```python
from build123d import *

# Parameters (mm, degrees)
ESQUISSE1_W        = 16
ESQUISSE1_H        = 28
BOSS_EXTRU_1_DEPTH = 6
BOSS_EXTRU_2_DEPTH = 0.5
CONG_1_R           = 0.5
ESQUISSE3_W        = 1
ESQUISSE3_H        = 4.650680728
BOSS_EXTRU_3_DEPTH = 0.5
ESQUISSE4_W        = 1
ESQUISSE4_H        = 3.990373045
BOSS_EXTRU_4_DEPTH = 0.5


with BuildPart() as part:
    # Esquisse1 → Boss.-Extru.1 (new body)
    with BuildSketch(Plane.XY):
        with Locations((2.66318356, 3.111111111)):
            Rectangle(ESQUISSE1_W, ESQUISSE1_H)
    extrude(amount=BOSS_EXTRU_1_DEPTH)

    # Esquisse2 → Boss.-Extru.2 (add)
    with BuildSketch(Plane.XY.offset(6)):
        with BuildLine():
            Line((-2.33681644, -0.888888889), (7.66318356, -0.888888889))
            ThreePointArc((7.66318356, -0.888888889), (8.370290341, -1.181782108), (8.66318356, -1.888888889))
            Line((8.66318356, -1.888888889), (8.66318356, -5.388888889))
            ThreePointArc((8.66318356, -5.388888889), (8.370290341, -6.09599567), (7.66318356, -6.388888889))
            Line((7.66318356, -6.388888889), (-2.33681644, -6.388888889))
            ThreePointArc((-2.33681644, -6.388888889), (-3.043923221, -6.09599567), (-3.33681644, -5.388888889))
            Line((-3.33681644, -5.388888889), (-3.33681644, -1.888888889))
            ThreePointArc((-3.33681644, -1.888888889), (-3.043923221, -1.181782108), (-2.33681644, -0.888888889))
        make_face()
    extrude(amount=BOSS_EXTRU_2_DEPTH)

    # Congé1
    cong_1_edges = [part.edges().sort_by_distance(p)[0] for p in [
        (-5.33681644, 17.111111111, 3),
        (10.66318356, 17.111111111, 3),
        (10.66318356, -10.888888889, 3),
        (-5.33681644, -10.888888889, 3),
    ]]
    fillet(cong_1_edges, radius=CONG_1_R)

    # Esquisse3 → Boss.-Extru.3 (add)
    with BuildSketch(Plane(origin=(0, 0, 0), x_dir=(-1, 0, 0), z_dir=(0, 0, -1))):
        with Locations((-0.244563406, 17.352420034)):
            Rectangle(ESQUISSE3_W, ESQUISSE3_H)
        with Locations((-3.244563406, 17.352420034)):
            Rectangle(ESQUISSE3_W, ESQUISSE3_H)
        with Locations((-6.244563406, 17.352420034)):
            Rectangle(ESQUISSE3_W, ESQUISSE3_H)
    extrude(amount=BOSS_EXTRU_3_DEPTH)

    # Esquisse4 → Boss.-Extru.4 (add)
    with BuildSketch(Plane(origin=(0, 0, 0), x_dir=(-1, 0, 0), z_dir=(0, 0, -1))):
        with Locations((-3.353859388, -10.762545732)):
            Rectangle(ESQUISSE4_W, ESQUISSE4_H)
    extrude(amount=BOSS_EXTRU_4_DEPTH)


solid = part.part
```
Check sheet for the modelled part. Datum: model origin and axes. Units: mm. A direction names the side the tool comes from. Coordinates: 2 decimals unless noted, no trailing zeros. Order: outer loops, then holes, each group sorted by start corner. A loop starts at its lowest first (then second) coordinate and runs counter-clockwise, first axis right, second up. Notation, with made-up numbers: M 62.25,36.5 L 80.25,36.5 A10 ccw 80.25,48.5 Z; hole C 55.5,23 d3. An arc over 180 degrees is marked long. One line per question, with ' | ' between items. Start each with the question number.
Item 1: Sectioned sample at B-B on x = 6.25. Record the cut outline in (y, z), and give its area (3 significant figures).
Item 2: Material ranges on line 1 (Z direction, x = 8.5, y = 5); line 2 (Z direction, x = 5.25, y = -6); line 3 (Y direction, x = -3.25, z = 5.75), recorded low to high.
Item 3: Access from +Z, -Z, +X, -X, +Y, -Y to the whole of each face (thin tool, end or side, straight path). Record for faces 1 (the flat face through (0, 18, 0)), 2 (the flat face through (3.4, -11.8, 0)), 3 (the cylindrical face through (8.378, -6.088, 6.246)).
Item 4: Gauge pin test, flat ends, axial feed: P1, Ø0.6, axis at y = 18, z = 0, coming from the +X side; P2, Ø1, axis at x = 5, z = 4.5, coming from the +Y side; P3, Ø1, axis at x = 3, z = 4, coming from the -Y side. Record the tip position at first contact, or that the pin passes through.
Item 5: Sectioned sample at A-A on y = -4.5. Record the cut outline in (x, z).
Item 6: Sectioned sample at D-D on y = 15.5. Record the cut outline in (x, z).
Item 7: Sectioned sample at C-C on z = 5.25. Record the cut outline in (x, y), and give its area (3 significant figures).
Answer below:
1) outline: M -10.89,0 L 15.03,0 L 15.03,-0.5 L 19.68,-0.5 L 19.68,0 L 17.11,0 L 17.11,6 L -0.89,6 L -0.89,6.5 L -6.39,6.5 L -6.39,6 L -10.89,6 Z | area: 173 mm^2
2) line 1: z = 0 to 6 | line 2: z = 0 to 6.5 | line 3: y = -10.89 to 17.11
3) face 1: +Z, +X, -X, +Y | face 2: +Z, +X, -X, -Y | face 3: +Z, +X, -Y
4) P1: stops at x = 6.74 | P2: stops at y = 17.11 | P3: stops at y = -10.89
5) outline: M -5.34,0 L 10.66,0 L 10.66,6 L 8.66,6 L 8.66,6.5 L -3.34,6.5 L -3.34,6 L -5.34,6 Z
6) outline: M -5.34,0 L -0.26,0 L -0.26,-0.5 L 0.74,-0.5 L 0.74,0 L 2.74,0 L 2.74,-0.5 L 3.74,-0.5 L 3.74,0 L 5.74,0 L 5.74,-0.5 L 6.74,-0.5 L 6.74,0 L 10.66,0 L 10.66,6 L -5.34,6 Z
7) outline: M -5.34,-10.39 A0.5 ccw -4.84,-10.89 L 10.16,-10.89 A0.5 ccw 10.66,-10.39 L 10.66,16.61 A0.5 ccw 10.16,17.11 L -4.84,17.11 A0.5 ccw -5.34,16.61 Z | area: 448 mm^2
